from build123d import *

# Parameters (mm, degrees)
BOSS_EXTRUDE1_DEPTH   = 0.8
SWEEP1_START          = -1.3
SWEEP1_DEPTH          = 2.6
SWEEP2_START          = -1.3
SWEEP2_DEPTH          = 2.6
CUT_EXTRUDE1_DEPTH    = 18.918364565
MIRROR3_COPY_1_DEPTH  = 18.918364565
SKETCH5_R             = 1.8
SKETCH5_R_2           = 1.2
BOSS_EXTRUDE2_DEPTH   = 0.8
M3X0_5_TAPPED_HOLE1_D = 2.5
FILLET1_R             = 0.2


# Read off the part's stored shape, not the designer's step: Sweep1, Sweep2
with BuildPart() as part:
    # Sketch1 → Boss-Extrude1 (new body)
    with BuildSketch(Plane(origin=(0, 0, 0), x_dir=(1, 0, 0), z_dir=(0, 1, 0))):
        with BuildLine():
            Line((-2.5, 2.85), (2.5, 2.85))
            ThreePointArc((2.5, 2.85), (2.78163021, 2.809523019), (3.040461339, 2.691368849))
            Line((3.040461339, 2.691368849), (4.959538661, 1.458631151))
            ThreePointArc((4.959538661, 1.458631151), (5.21836979, 1.340476981), (5.5, 1.3))
            Line((5.5, 1.3), (5.5, -1.3))
            ThreePointArc((5.5, -1.3), (5.21836979, -1.340476981), (4.959538661, -1.458631151))
            Line((4.959538661, -1.458631151), (3.040461339, -2.691368849))
            ThreePointArc((3.040461339, -2.691368849), (2.78163021, -2.809523019), (2.5, -2.85))
            Line((2.5, -2.85), (-2.5, -2.85))
            ThreePointArc((-2.5, -2.85), (-2.78163021, -2.809523019), (-3.040461339, -2.691368849))
            Line((-3.040461339, -2.691368849), (-4.959538661, -1.458631151))
            ThreePointArc((-4.959538661, -1.458631151), (-5.21836979, -1.340476981), (-5.5, -1.3))
            Line((-5.5, -1.3), (-5.5, 1.3))
            ThreePointArc((-5.5, 1.3), (-5.21836979, 1.340476981), (-4.959538661, 1.458631151))
            Line((-4.959538661, 1.458631151), (-3.040461339, 2.691368849))
            ThreePointArc((-3.040461339, 2.691368849), (-2.78163021, 2.809523019), (-2.5, 2.85))
        make_face()
    extrude(amount=-BOSS_EXTRUDE1_DEPTH)

    # Sweep1 outline → Sweep1 (add)
    with BuildSketch(Plane.XY.offset(SWEEP1_START)):
        with BuildLine():
            Line((-13.071251863, -1.626643489), (-17.169047305, -3.537476885))
            Line((-17.169047305, -3.537476885), (-16.830952695, -4.262523115))
            Line((-16.830952695, -4.262523115), (-12.733157253, -2.351689719))
            ThreePointArc((-12.733157253, -2.351689719), (-12.619409099, -2.313077423), (-12.5, -2.3))
            Line((-12.5, -2.3), (-10.5, -2.3))
            ThreePointArc((-10.5, -2.3), (-10.110231056, -2.259075901), (-9.737462135, -2.138088534))
            Line((-9.737462135, -2.138088534), (-6.937462135, -0.892887369))
            ThreePointArc((-6.937462135, -0.892887369), (-6.723607459, -0.823477842), (-6.5, -0.8))
            Line((-6.5, -0.8), (-5.5, -0.8))
            Line((-5.5, -0.8), (-5.5, 0))
            Line((-5.5, 0), (-6.5, 0))
            ThreePointArc((-6.5, 0), (-6.889768944, -0.040924099), (-7.262537865, -0.161911466))
            Line((-7.262537865, -0.161911466), (-10.062537865, -1.407112631))
            ThreePointArc((-10.062537865, -1.407112631), (-10.276392541, -1.476522158), (-10.5, -1.5))
            Line((-10.5, -1.5), (-12.5, -1.5))
            ThreePointArc((-12.5, -1.5), (-12.79256079, -1.532040618), (-13.071251863, -1.626643489))
        make_face()
    extrude(amount=SWEEP1_DEPTH)

    # Sweep2 outline → Sweep2 (add)
    with BuildSketch(Plane.XY.offset(SWEEP2_START)):
        with BuildLine():
            ThreePointArc((13.071251863, -1.626643489), (12.79256079, -1.532040618), (12.5, -1.5))
            Line((12.5, -1.5), (10.5, -1.5))
            ThreePointArc((10.5, -1.5), (10.276392541, -1.476522158), (10.062537865, -1.407112631))
            Line((10.062537865, -1.407112631), (7.262537865, -0.161911466))
            ThreePointArc((7.262537865, -0.161911466), (6.889768944, -0.040924099), (6.5, 0))
            Line((6.5, 0), (5.5, 0))
            Line((5.5, 0), (5.5, -0.8))
            Line((5.5, -0.8), (6.5, -0.8))
            ThreePointArc((6.5, -0.8), (6.723607459, -0.823477842), (6.937462135, -0.892887369))
            Line((6.937462135, -0.892887369), (9.737462135, -2.138088534))
            ThreePointArc((9.737462135, -2.138088534), (10.110231056, -2.259075901), (10.5, -2.3))
            Line((10.5, -2.3), (12.5, -2.3))
            ThreePointArc((12.5, -2.3), (12.619409099, -2.313077423), (12.733157253, -2.351689719))
            Line((12.733157253, -2.351689719), (16.830952695, -4.262523115))
            Line((16.830952695, -4.262523115), (17.169047305, -3.537476885))
            Line((17.169047305, -3.537476885), (13.071251863, -1.626643489))
        make_face()
    extrude(amount=SWEEP2_DEPTH)

    # Sketch3 → Cut-Extrude1 (cut, through all)
    with BuildSketch(Plane(origin=(0, 0, 0), x_dir=(1, 0, 0), z_dir=(0, 1, 0))):
        with BuildLine():
            Line((-17.169047305, 0.75), (-16.369047305, 0.75))
            ThreePointArc((-16.369047305, 0.75), (-16.335739791, 0.752792978), (-16.303362548, 0.761093905))
            Line((-16.303362548, 0.761093905), (-14.833259195, 1.272265238))
            ThreePointArc((-14.833259195, 1.272265238), (-14.75231609, 1.293017555), (-14.669047305, 1.3))
            Line((-14.669047305, 1.3), (-17.169047305, 1.3))
            Line((-17.169047305, 1.3), (-17.169047305, 0.75))
        make_face()
    cut_extrude1 = extrude(amount=-CUT_EXTRUDE1_DEPTH, mode=Mode.SUBTRACT)

    # Mirror1: Cut-Extrude1 across plane
    add(cut_extrude1.mirror(Plane.XY), mode=Mode.SUBTRACT)

    # Mirror3: Cut-Extrude1 across plane
    add(cut_extrude1.mirror(Plane(origin=(0, 0, 0), x_dir=(0, 0, 1), z_dir=(1, 0, 0))), mode=Mode.SUBTRACT)

    # Mirror3 copy 1 sketch → Mirror3 copy 1 (cut, through all)
    with BuildSketch(Plane(origin=(0, 0, 0), x_dir=(-1, 0, 0), z_dir=(0, 1, 0))):
        with BuildLine():
            Line((-17.169047305, 0.75), (-16.369047305, 0.75))
            ThreePointArc((-16.369047305, 0.75), (-16.335739791, 0.752792978), (-16.303362548, 0.761093905))
            Line((-16.303362548, 0.761093905), (-14.833259195, 1.272265238))
            ThreePointArc((-14.833259195, 1.272265238), (-14.75231609, 1.293017555), (-14.669047305, 1.3))
            Line((-14.669047305, 1.3), (-17.169047305, 1.3))
            Line((-17.169047305, 1.3), (-17.169047305, 0.75))
        make_face()
    extrude(amount=-MIRROR3_COPY_1_DEPTH, mode=Mode.SUBTRACT)

    # Sketch5 → Boss-Extrude2 (add)
    with BuildSketch(Plane(origin=(0, 0, 0), x_dir=(1, 0, 0), z_dir=(0, 1, 0))):
        with Locations(Location((0, 0, 0), (0, 0, 270))):
            Circle(SKETCH5_R)
        with Locations(Location((0, 0, 0), (0, 0, 270))):
            Circle(SKETCH5_R_2, mode=Mode.SUBTRACT)
    extrude(amount=BOSS_EXTRUDE2_DEPTH)

    # M3x0.5 Tapped Hole1 (through all)
    with Locations(Plane(origin=(0, 0.8, 0), x_dir=(1, 0, 0), z_dir=(0, 1, 0))):
        with Locations((0, 0)):
            Hole(M3X0_5_TAPPED_HOLE1_D / 2)

    # Fillet1
    fillet1_edges = [part.edges().sort_by_distance(p)[0] for p in [
        (-17, -3.9, -0.75),
        (-17, -3.9, 0.75),
        (17, -3.9, -0.75),
        (17, -3.9, 0.75),
    ]]
    fillet(fillet1_edges, radius=FILLET1_R)


solid = part.part
Work out the finished part from the listing and answer in its coordinate system (mm). A direction names the side the tool comes from. Give positions to 0.01 mm unless a question says otherwise; leave off trailing zeros. Loops run counter-clockwise (first coordinate to the right, second up) from the corner with the lowest first, then second, coordinate; pieces in that order, holes last. Notation, with made-up numbers: (-10, 70.5) -> (42, 70.5) arc R26 ccw to (42, 99.5) -> close; hole circle Ø9 at (-31, 72.5). An arc over 180 degrees is marked (long way). Use a Markdown table: item, result. Add a question column.
1) The part is cut by section B-B, the plane x = -13.5. Determine the outline of the cut face in (y, z).
2) Consider line 1 along Y through (x, z) = (-3, 1.2); line 2 along Z through (x, y) = (0, -0.15); line 3 along X through (y, z) = (-0.4, -0.5). Determine where each line is inside the solid, lowest interval first.
3) The part is cut by section A-A, the plane x = 0. Determine the outline of the cut face in (y, z), plus the area to 3 significant figures.
4) Which of the six approach directions +Z, -Z, +X, -X, +Y, -Y give full straight-line access (tool end or side, diameter ignored) to faces 4 (the flat face through (-10, -2, 1.3)), 5 (the cylindrical face through (-0.689, 0.394, 1.663)), 6 (the flat face through (14.75, -3.29, -0.02)), 7 (the flat face through (10, -2, 1.3)), 8 (the flat face through (10, -2, -1.3))?
5) Each of these flat-tipped pins is pushed along its axis until it touches: P1, Ø2, axis at x = -9.5, z = 0, coming from the +Y side; P2, Ø3, axis at y = -0.5, z = -1.5, coming from the -X side; P3, Ø1, axis at x = -11.5, z = 0.5, coming from the +Y side. Where does it stop, or does it pass through?
6) For a pull along X with two mould halves and no side action, classify faces 1 (the flat face through (11, -2.3, 0)), 2 (the flat face through (-10, -2, -1.3)), 3 (the flat face through (15.579, -3.221, -1.013)) as +X half, -X half, draft (parallel to the pull), parting line (faces both ways), or undercut.
Reported:
| question | item | result |
|---|---|---|
| 1 | outline | (-2.71, -1.3) -> (-1.83, -1.3) -> (-1.83, 1.3) -> (-2.71, 1.3) -> close |
| 2 | line 1 | y = -0.8 to 0 |
| 2 | line 2 | z = -2.85 to -1.25, 1.25 to 2.85 |
| 2 | line 3 | x = -7.8 to -1.15, 1.15 to 7.8 |
| 3 | outline | (-0.8, -2.85) -> (0, -2.85) -> (0, -1.8) -> (0.8, -1.8) -> (0.8, -1.25) -> (-0.8, -1.25) -> close; (-0.8, 1.25) -> (0.8, 1.25) -> (0.8, 1.8) -> (0, 1.8) -> (0, 2.85) -> (-0.8, 2.85) -> close |
| 3 | area | 3.44 mm^2 |
| 4 | face 4 | +Z, -X, +Y, -Y |
| 4 | face 5 | +Y |
| 4 | face 6 | +Z, -Z, -Y |
| 4 | face 7 | +Z, +X, +Y, -Y |
| 4 | face 8 | -Z, +X, +Y, -Y |
| 5 | P1 | stops at y = -0.71 |
| 5 | P2 | stops at x = -13.84 |
| 5 | P3 | stops at y = -1.5 |
| 6 | face 1 | undercut |
| 6 | face 2 | draft |
| 6 | face 3 | +X half |
